Model file for the job. Use its own axes, mm. A direction names the side the tool comes from. Coordinates: 2 decimals unless noted, no trailing zeros. Order: outer loops, then holes, each group sorted by start corner. A loop starts at its lowest first (then second) coordinate and runs counter-clockwise, first axis right, second up. Notation, with made-up numbers: (-38.75, 2) -> (-15.75, 2) arc R26 ccw to (-15.75, 34) -> close; hole circle Ø3 at (-14, 64.25). An arc over 180 degrees is marked (long way). Return JSON: item names as keys, results as strings. Group by question number.
1) Pull direction X, two halves, no side cores. Call faces 1 (the flat face through (4, 21, 2)), 2 (the cylindrical face through (-45.99, 0.96, 1.97)), 3 (the flat face through (0, -45.826, 2)), 4 (the cylindrical face through (-28.994, -0.582, 1.972)): +X half, -X half, draft (parallel to the pull), parting line (faces both ways), or undercut.
2) Probe line 1 (X direction, y = -0.5, z = 33.5); line 2 (Z direction, x = 1, y = 19); line 3 (X direction, y = 10, z = 6). List the from-to ranges inside material, lowest first.
3) Cut at A-A (x = 0). State how many separate pieces and enclosed holes the cut face has, and give its area (3 significant figures).
4) Cut at B-B (z = 28). Write the cut outline in (x, y), and give its area (3 significant figures).
5) Flat gauge pins, fed straight in: pin 1 (1.6 mm diameter, centred on y = -43.5, z = 3, fed in from +X); pin 2 (10 mm diameter, centred on y = -10, z = 16, fed in from +X); pin 3 (4.5 mm diameter, centred on y = 22.5, z = 2.5, fed in from +X); pin 4 (1.5 mm diameter, centred on x = 18, z = 5.5, fed in from +Y). Where does each tip first touch, or does it go through?
6) Which spindle directions (+Z, -Z, +X, -X, +Y, -Y) get a long thin tool onto all of the face, cutting with end or side? Do faces 5 (the flat face through (10, -10, 0)), 6 (the flat face through (-4, -21, 2)). Say none if no direction does.
from build123d import *

# Parameters (mm, degrees)
F1_DEPTH = 40
F2_DEPTH = 4


with BuildPart() as f1:
    # F0 (on Top) → F1 (new body)
    with BuildSketch(Plane.XY):
        with BuildLine():
            ThreePointArc((4, 12.2115723803), (10.4048666498, 7.5406398933), (12.85, 0))
            ThreePointArc((12.85, 0), (10.4048666498, -7.5406398933), (4, -12.2115723803))
            Line((4, -12.2115723803), (4, -13.9373598648))
            ThreePointArc((4, -13.9373598648), (11.5812348219, -8.7249641833), (14.5, 0))
            ThreePointArc((14.5, 0), (11.5812348219, 8.7249641833), (4, 13.9373598648))
            Line((4, 13.9373598648), (4, 12.2115723803))
        make_face()
        with BuildLine():
            ThreePointArc((-4, 12.2115723803), (0, 12.85), (4, 12.2115723803))
            Line((4, 12.2115723803), (4, 13.9373598648))
            ThreePointArc((4, 13.9373598648), (0, 14.5), (-4, 13.9373598648))
            Line((-4, 13.9373598648), (-4, 12.2115723803))
        make_face()
        with BuildLine():
            Line((4, -13.9373598648), (4, -12.2115723803))
            ThreePointArc((4, -12.2115723803), (0, -12.85), (-4, -12.2115723803))
            Line((-4, -12.2115723803), (-4, -13.9373598648))
            ThreePointArc((-4, -13.9373598648), (0, -14.5), (4, -13.9373598648))
        make_face()
        with BuildLine():
            ThreePointArc((-4, -12.2115723803), (-12.85, 0), (-4, 12.2115723803))
            Line((-4, 12.2115723803), (-4, 13.9373598648))
            ThreePointArc((-4, 13.9373598648), (-14.5, 0), (-4, -13.9373598648))
            Line((-4, -13.9373598648), (-4, -12.2115723803))
        make_face()
    extrude(amount=F1_DEPTH)

    # F0 (on Top) → F2 (join)
    with BuildSketch(Plane.XY):
        with BuildLine():
            Line((4, -28.7228132327), (4, -13.9373598648))
            ThreePointArc((4, -13.9373598648), (0, -14.5), (-4, -13.9373598648))
            Line((-4, -13.9373598648), (-4, -28.7228132327))
            ThreePointArc((-4, -28.7228132327), (0, -29), (4, -28.7228132327))
        make_face()
        with BuildLine():
            ThreePointArc((-4, 40.3019850628), (0, 40.5), (4, 40.3019850628))
            Line((4, 40.3019850628), (4, 42.3113459961))
            ThreePointArc((4, 42.3113459961), (0, 42.5), (-4, 42.3113459961))
            Line((-4, 42.3113459961), (-4, 40.3019850628))
        make_face()
        with BuildLine():
            ThreePointArc((-4, -40.3019850628), (-40.5, 0), (-4, 40.3019850628))
            Line((-4, 40.3019850628), (-4, 42.3113459961))
            ThreePointArc((-4, 42.3113459961), (-42.5, 0), (-4, -42.3113459961))
            Line((-4, -42.3113459961), (-4, -40.3019850628))
        make_face()
        with BuildLine():
            Line((4, -42.3113459961), (4, -40.3019850628))
            ThreePointArc((4, -40.3019850628), (0, -40.5), (-4, -40.3019850628))
            Line((-4, -40.3019850628), (-4, -42.3113459961))
            ThreePointArc((-4, -42.3113459961), (0, -42.5), (4, -42.3113459961))
        make_face()
        with BuildLine():
            Line((4, 42.3113459961), (4, 40.3019850628))
            ThreePointArc((4, 40.3019850628), (30.0187441443, 27.1868534406), (40.5, 0))
            ThreePointArc((40.5, 0), (30.0187441443, -27.1868534406), (4, -40.3019850628))
            Line((4, -40.3019850628), (4, -42.3113459961))
            ThreePointArc((4, -42.3113459961), (31.434455618, -28.6028844699), (42.5, 0))
            ThreePointArc((42.5, 0), (31.434455618, 28.6028844699), (4, 42.3113459961))
        make_face()
        with BuildLine():
            ThreePointArc((-4, 37.7888872554), (0, 38), (4, 37.7888872554))
            Line((4, 37.7888872554), (4, 39.7994974843))
            ThreePointArc((4, 39.7994974843), (0, 40), (-4, 39.7994974843))
            Line((-4, 39.7994974843), (-4, 37.7888872554))
        make_face()
        with BuildLine():
            ThreePointArc((-4, -37.7888872554), (-38, 0), (-4, 37.7888872554))
            Line((-4, 37.7888872554), (-4, 39.7994974843))
            ThreePointArc((-4, 39.7994974843), (-40, 0), (-4, -39.7994974843))
            Line((-4, -39.7994974843), (-4, -37.7888872554))
        make_face()
        with BuildLine():
            Line((4, -39.7994974843), (4, -37.7888872554))
            ThreePointArc((4, -37.7888872554), (0, -38), (-4, -37.7888872554))
            Line((-4, -37.7888872554), (-4, -39.7994974843))
            ThreePointArc((-4, -39.7994974843), (0, -40), (4, -39.7994974843))
        make_face()
        with BuildLine():
            Line((4, 39.7994974843), (4, 37.7888872554))
            ThreePointArc((4, 37.7888872554), (28.2488937837, 25.4165300543), (38, 0))
            ThreePointArc((38, 0), (28.2488937837, -25.4165300543), (4, -37.7888872554))
            Line((4, -37.7888872554), (4, -39.7994974843))
            ThreePointArc((4, -39.7994974843), (29.6647939484, -26.83281573), (40, 0))
            ThreePointArc((40, 0), (29.6647939484, 26.83281573), (4, 39.7994974843))
        make_face()
        with BuildLine():
            Line((4, -40.3019850628), (4, -39.7994974843))
            ThreePointArc((4, -39.7994974843), (0, -40), (-4, -39.7994974843))
            Line((-4, -39.7994974843), (-4, -40.3019850628))
            ThreePointArc((-4, -40.3019850628), (0, -40.5), (4, -40.3019850628))
        make_face()
        with BuildLine():
            Line((4, -44.3198601081), (4, -42.3113459961))
            ThreePointArc((4, -42.3113459961), (0, -42.5), (-4, -42.3113459961))
            Line((-4, -42.3113459961), (-4, -44.3198601081))
            ThreePointArc((-4, -44.3198601081), (0, -44.5), (4, -44.3198601081))
        make_face()
        with BuildLine():
            ThreePointArc((-4, -44.3198601081), (-44.5, 0), (-4, 44.3198601081))
            Line((-4, 44.3198601081), (-4, 45.8257569496))
            ThreePointArc((-4, 45.8257569496), (-46, 0), (-4, -45.8257569496))
            Line((-4, -45.8257569496), (-4, -44.3198601081))
        make_face()
        with BuildLine():
            Line((4, 45.8257569496), (4, 44.3198601081))
            ThreePointArc((4, 44.3198601081), (32.8500380517, 30.0187441443), (44.5, 0))
            ThreePointArc((44.5, 0), (32.8500380517, -30.0187441443), (4, -44.3198601081))
            Line((4, -44.3198601081), (4, -45.8257569496))
            ThreePointArc((4, -45.8257569496), (33.9116499156, -31.0805405358), (46, 0))
            ThreePointArc((46, 0), (33.9116499156, 31.0805405358), (4, 45.8257569496))
        make_face()
        with BuildLine():
            ThreePointArc((-4, 44.3198601081), (0, 44.5), (4, 44.3198601081))
            Line((4, 44.3198601081), (4, 45.8257569496))
            Line((4, 45.8257569496), (-4, 45.8257569496))
            Line((-4, 45.8257569496), (-4, 44.3198601081))
        make_face()
        with BuildLine():
            Line((4, -45.8257569496), (4, -44.3198601081))
            ThreePointArc((4, -44.3198601081), (0, -44.5), (-4, -44.3198601081))
            Line((-4, -44.3198601081), (-4, -45.8257569496))
            Line((-4, -45.8257569496), (4, -45.8257569496))
        make_face()
        with BuildLine():
            ThreePointArc((-4, -34.7706773014), (-35, 0), (-4, 34.7706773014))
            Line((-4, 34.7706773014), (-4, 36.7831483155))
            ThreePointArc((-4, 36.7831483155), (-37, 0), (-4, -36.7831483155))
            Line((-4, -36.7831483155), (-4, -34.7706773014))
        make_face()
        with BuildLine():
            ThreePointArc((-4, -31.7490157328), (-32, 0), (-4, 31.7490157328))
            Line((-4, 31.7490157328), (-4, 33.7638860323))
            ThreePointArc((-4, 33.7638860323), (-34, 0), (-4, -33.7638860323))
            Line((-4, -33.7638860323), (-4, -31.7490157328))
        make_face()
        with BuildLine():
            ThreePointArc((-4, -28.7228132327), (-29, 0), (-4, 28.7228132327))
            Line((-4, 28.7228132327), (-4, 30.7408522979))
            ThreePointArc((-4, 30.7408522979), (-31, 0), (-4, -30.7408522979))
            Line((-4, -30.7408522979), (-4, -28.7228132327))
        make_face()
        with BuildLine():
            Line((4, 36.7831483155), (4, 34.7706773014))
            ThreePointArc((4, 34.7706773014), (26.1247009552, 23.2916293977), (35, 0))
            ThreePointArc((35, 0), (26.1247009552, -23.2916293977), (4, -34.7706773014))
            Line((4, -34.7706773014), (4, -36.7831483155))
            ThreePointArc((4, -36.7831483155), (27.5408787078, -24.7082982012), (37, 0))
            ThreePointArc((37, 0), (27.5408787078, 24.7082982012), (4, 36.7831483155))
        make_face()
        with BuildLine():
            Line((4, 33.7638860323), (4, 31.7490157328))
            ThreePointArc((4, 31.7490157328), (24, 21.1660104885), (32, 0))
            ThreePointArc((32, 0), (24, -21.1660104885), (4, -31.7490157328))
            Line((4, -31.7490157328), (4, -33.7638860323))
            ThreePointArc((4, -33.7638860323), (25.4165300543, -22.5831795813), (34, 0))
            ThreePointArc((34, 0), (25.4165300543, 22.5831795813), (4, 33.7638860323))
        make_face()
        with BuildLine():
            Line((4, 30.7408522979), (4, 28.7228132327))
            ThreePointArc((4, 28.7228132327), (21.8746428542, 19.0394327647), (29, 0))
            ThreePointArc((29, 0), (21.8746428542, -19.0394327647), (4, -28.7228132327))
            Line((4, -28.7228132327), (4, -30.7408522979))
            ThreePointArc((4, -30.7408522979), (23.2916293977, -20.4572725455), (31, 0))
            ThreePointArc((31, 0), (23.2916293977, 20.4572725455), (4, 30.7408522979))
        make_face()
        with BuildLine():
            ThreePointArc((-4, 28.7228132327), (0, 29), (4, 28.7228132327))
            Line((4, 28.7228132327), (4, 30.7408522979))
            ThreePointArc((4, 30.7408522979), (0, 31), (-4, 30.7408522979))
            Line((-4, 30.7408522979), (-4, 28.7228132327))
        make_face()
        with BuildLine():
            ThreePointArc((-4, 31.7490157328), (0, 32), (4, 31.7490157328))
            Line((4, 31.7490157328), (4, 33.7638860323))
            ThreePointArc((4, 33.7638860323), (0, 34), (-4, 33.7638860323))
            Line((-4, 33.7638860323), (-4, 31.7490157328))
        make_face()
        with BuildLine():
            ThreePointArc((-4, 34.7706773014), (0, 35), (4, 34.7706773014))
            Line((4, 34.7706773014), (4, 36.7831483155))
            ThreePointArc((4, 36.7831483155), (0, 37), (-4, 36.7831483155))
            Line((-4, 36.7831483155), (-4, 34.7706773014))
        make_face()
        with BuildLine():
            Line((4, -30.7408522979), (4, -28.7228132327))
            ThreePointArc((4, -28.7228132327), (0, -29), (-4, -28.7228132327))
            Line((-4, -28.7228132327), (-4, -30.7408522979))
            ThreePointArc((-4, -30.7408522979), (0, -31), (4, -30.7408522979))
        make_face()
        with BuildLine():
            Line((4, -33.7638860323), (4, -31.7490157328))
            ThreePointArc((4, -31.7490157328), (0, -32), (-4, -31.7490157328))
            Line((-4, -31.7490157328), (-4, -33.7638860323))
            ThreePointArc((-4, -33.7638860323), (0, -34), (4, -33.7638860323))
        make_face()
        with BuildLine():
            Line((4, -36.7831483155), (4, -34.7706773014))
            ThreePointArc((4, -34.7706773014), (0, -35), (-4, -34.7706773014))
            Line((-4, -34.7706773014), (-4, -36.7831483155))
            ThreePointArc((-4, -36.7831483155), (0, -37), (4, -36.7831483155))
        make_face()
        with BuildLine():
            Line((4, -31.7490157328), (4, -30.7408522979))
            ThreePointArc((4, -30.7408522979), (0, -31), (-4, -30.7408522979))
            Line((-4, -30.7408522979), (-4, -31.7490157328))
            ThreePointArc((-4, -31.7490157328), (0, -32), (4, -31.7490157328))
        make_face()
        with BuildLine():
            Line((4, -34.7706773014), (4, -33.7638860323))
            ThreePointArc((4, -33.7638860323), (0, -34), (-4, -33.7638860323))
            Line((-4, -33.7638860323), (-4, -34.7706773014))
            ThreePointArc((-4, -34.7706773014), (0, -35), (4, -34.7706773014))
        make_face()
        with BuildLine():
            Line((4, -37.7888872554), (4, -36.7831483155))
            ThreePointArc((4, -36.7831483155), (0, -37), (-4, -36.7831483155))
            Line((-4, -36.7831483155), (-4, -37.7888872554))
            ThreePointArc((-4, -37.7888872554), (0, -38), (4, -37.7888872554))
        make_face()
        with BuildLine():
            ThreePointArc((-4, 13.9373598648), (0, 14.5), (4, 13.9373598648))
            Line((4, 13.9373598648), (4, 28.7228132327))
            ThreePointArc((4, 28.7228132327), (0, 29), (-4, 28.7228132327))
            Line((-4, 28.7228132327), (-4, 13.9373598648))
        make_face()
    extrude(amount=F2_DEPTH)


solid = f1.part
Answers below:
{
 "1": {"face 1": "undercut", "face 2": "-X half", "face 3": "draft", "face 4": "undercut"},
 "2": {"line 1": "x = -14.49 to -12.84, 12.84 to 14.49", "line 2": "z = 0 to 4", "line 3": "x = -10.5 to -8.07, 8.07 to 10.5"},
 "3": {"separate pieces": "7", "enclosed holes": "0", "area": "361 mm^2"},
 "4": {"outline": "circle Ø29 at (0, 0); hole circle Ø25.7 at (0, 0)", "area": "142 mm^2"},
 "5": {"pin 1": "stops at x = 17.11", "pin 2": "stops at x = 13.61", "pin 3": "stops at x = 41.3", "pin 4": "passes through"},
 "6": {"face 5": "-Z, +X, -X, +Y, -Y", "face 6": "+Z, -Z"}
}
